from build123d import *

# Parameters (mm, degrees)
BOSS_EXTRUDE1_DEPTH      = 141
BOSS_EXTRUDE1_DEPTH_BACK = 141
CAVITY1_START            = -2
CAVITY1_OUTLINE_W        = 282
CAVITY1_OUTLINE_H        = 40
CAVITY1_DEPTH            = 2


# Read off the part's stored shape, not the designer's step: Cavity1
with BuildPart() as part:
    # Sketch1 → Boss-Extrude1 (new, two sides: drawn at the far end of the back side and taken through both)
    with BuildSketch(Plane(origin=(0, 0, 0), x_dir=(0, 0, -1), z_dir=(1, 0, 0)).offset(-BOSS_EXTRUDE1_DEPTH_BACK)):
        with BuildLine():
            Line((12, -285), (-10, -285))
            Line((-10, -285), (-10, -330.531793911))
            ThreePointArc((-10, -330.531793911), (-8.870108332, -335.149280044), (-5.735764364, -338.723314354))
            Line((-5.735764364, -338.723314354), (26.861841993, -361.548404053))
            Line((26.861841993, -361.548404053), (31.450453484, -354.995187698))
            Line((31.450453484, -354.995187698), (6.875892155, -337.787894608))
            Line((6.875892155, -337.787894608), (8.023045028, -336.149590519))
            Line((8.023045028, -336.149590519), (32.597606357, -353.35688361))
            Line((32.597606357, -353.35688361), (36.795346904, -347.361888815))
            Line((36.795346904, -347.361888815), (16.264235636, -332.985849937))
            ThreePointArc((16.264235636, -332.985849937), (13.129891668, -329.411815627), (12, -324.794329494))
            Line((12, -324.794329494), (12, -285))
        make_face()
    extrude(amount=BOSS_EXTRUDE1_DEPTH + BOSS_EXTRUDE1_DEPTH_BACK)

    # Cavity1 outline → Cavity1 (cut)
    with BuildSketch(Plane.XY.offset(CAVITY1_START)):
        with Locations((0, -305)):
            Rectangle(CAVITY1_OUTLINE_W, CAVITY1_OUTLINE_H)
    extrude(amount=CAVITY1_DEPTH, mode=Mode.SUBTRACT)


solid = part.part
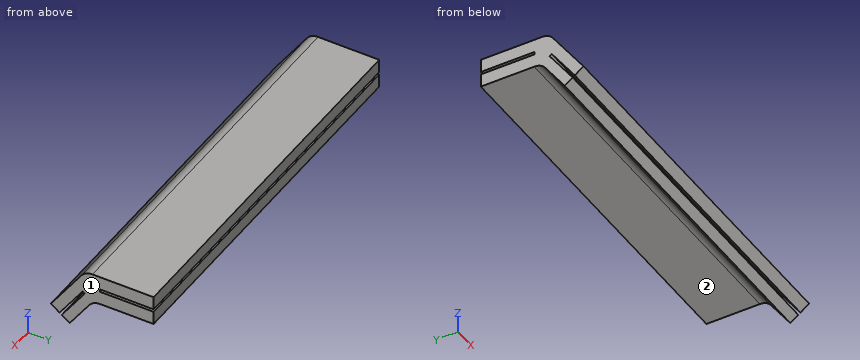
Verification items for the finished model (mm, model axes). Face numbers are marked on the shaded views. A direction names the side the tool comes from. Round coordinates to 2 decimals unless told otherwise and drop trailing zeros. Loops run counter-clockwise (first coordinate to the right, second up) from the corner with the lowest first, then second, coordinate; pieces in that order, holes last. Notation, with made-up numbers: (37.25, -3.5) - (76.25, -3.5) arc R21 cw to (76.25, 32.5) - close; hole circle Ø6 at (4, 77). An arc over 180 degrees is marked (long way). Answer in a Markdown table with one row per item. Add a question column.
Q1. Section check A-A on y = -321.5. Enter the section's corners in (x, z), plus the area to 3 significant figures.
Q2. Gauge pin test, flat ends, axial feed: pin 1 (20 mm diameter, centred on x = 57.5, y = -303.5, fed in from -Z); pin 2 (1 mm diameter, centred on x = 59, y = -341.5, fed in from +Z); pin 3 (1 mm diameter, centred on x = 66.5, z = -1, fed in from +Y); pin 4 (6 mm diameter, centred on y = -337, z = -8, fed in from +X). Record the tip position at first contact, or that the pin passes through.
Q3. Material ranges on line 1 (Z direction, x = 100, y = -313); line 2 (Y direction, x = -91.5, z = -23); line 3 (Y direction, x = -111, z = -18), recorded low to high.
Q4. Section check B-B on x = -80. Enter the section's corners in (y, z), plus the area to 3 significant figures.
Q5. Tool access check on the marked faces 1 and 2. Record the directions out of +Z, -Z, +X, -X, +Y, -Y that give a thin tool (end or side, any length) a straight path to the whole face; none if there is none.
Found:
| question | item | result |
|---|---|---|
| 1 | outline | (-141, -12) - (141, -12) - (141, -2) - (-141, -2) - close; (-141, 0) - (141, 0) - (141, 10) - (-141, 10) - close |
| 1 | area | 5,640 mm² |
| 2 | pin 1 | stops at z = -12 |
| 2 | pin 2 | stops at z = 2.48 |
| 2 | pin 3 | stops at y = -325 |
| 2 | pin 4 | stops at x = 141 |
| 3 | line 1 | z = -12 to -2, 0 to 10 |
| 3 | line 2 | y = -358.84 to -349.08, -346.64 to -337.7 |
| 3 | line 3 | y = -355.34 to -345.58, -343.14 to -334.2 |
| 4 | outline | (-361.55, -26.86) - (-355, -31.45) - (-337.79, -6.88) - (-336.15, -8.02) - (-353.36, -32.6) - (-347.36, -36.8) - (-332.99, -16.26) arc R10 cw to (-324.79, -12) - (-285, -12) - (-285, -2) - (-325, -2) - (-325, 0) - (-285, 0) - (-285, 10) - (-330.53, 10) arc R10 ccw to (-338.72, 5.74) - close |
| 4 | area | 1,560 mm² |
| 5 | face 1 | +Z, -Z, +X, +Y, -Y |
| 5 | face 2 | -Z, +X, -X, +Y |
